Part model, mm, in its own coordinate system. Face numbers are marked on the shaded views. A direction names the side the tool comes from. Give positions to 0.01 mm unless a question says otherwise; leave off trailing zeros. Order: outer loops, then holes, each group sorted by start corner. A loop starts at its lowest first (then second) coordinate and runs counter-clockwise, first axis right, second up. Notation, with made-up numbers: M 4.5,67.5 L 45.5,67.5 A26 ccw 45.5,99.5 Z; hole C 88.5,74.5 d6. An arc over 180 degrees is marked long. One line per question, with ' | ' between items.
Autodesk Inventor part; units mm, degrees
ref_plane "YZ Plane" through (0, 0, 0) normal (1, 0, 0) x (0, 1, 0)
ref_plane "XZ Plane" through (0, 0, 0) normal (0, 1, 0) x (-1, 0, 0)
ref_plane "XY Plane" through (0, 0, 0) normal (0, 0, 1) x (1, 0, 0)
sketch "Sketch1" plane through (0, 0, 0) normal (0, 0, 1) x (1, 0, 0)
  arc A0 (-2.8807, 19.6399) -> (-2.8807, -19.6399) centre (0, 0) ccw
  arc A1 (131.6255, -39.3688) -> (131.6255, 39.3688) centre (137.4, 0) ccw
  line L0 (0, 0) -> (137.4, 0)
  line L1 (0, 0) -> (137.4, 0) construction
  line L2 (-2.8807, 19.6399) -> (131.6255, 39.3688)
  line L3 (-2.8807, -19.6399) -> (131.6255, -39.3688)
  arc A2 (131.9303, -37.291) -> (131.9303, 37.291) centre (137.4, 0) ccw
  line L4 (131.9303, 37.291) -> (-2.5759, 17.5621)
  arc A3 (-2.5759, 17.5621) -> (-2.5759, -17.5621) centre (0, 0) ccw
  line L5 (-2.5759, -17.5621) -> (131.9303, -37.291)
  arc A4 (131.4078, -40.8529) -> (131.4078, 40.8529) centre (137.4, 0) ccw
  line L6 (131.4078, 40.8529) -> (-3.0984, 21.124)
  arc A5 (-3.0984, 21.124) -> (-3.0984, -21.124) centre (0, 0) ccw
  line L7 (-3.0984, -21.124) -> (131.4078, -40.8529)
  dimension "d0" = 39.7
  dimension "d1" = 79.58
  dimension "d2" = 137.4
  dimension "d3" = 0
  dimension "d4" = 2.1
  dimension "d5" = 1.5
extrude "Extrusion1" add sketch "Sketch1" along normal blind 15 contours L2 A1 L3 A0 | L7 A5 L6 A4
properties part number "HTD5M 93 Belt" material "Rubber"
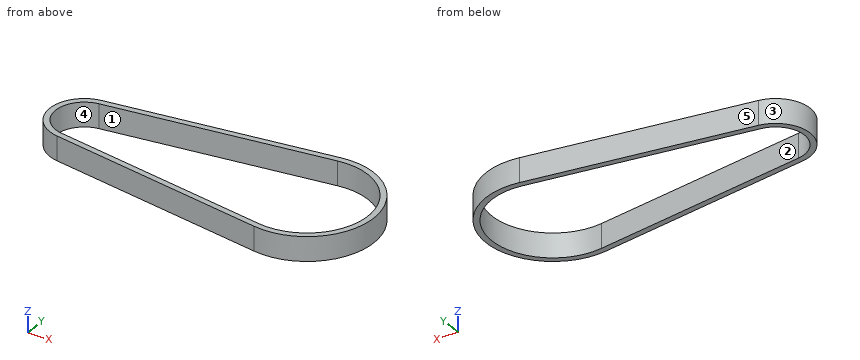
1. Slice it at A-A on x = 137.4. Give the cut face in (y, z), then the cut area to 3 significant figures.
Worked out:
outline: M -41.29,0 L -37.69,0 L -37.69,15 L -41.29,15 Z; M 37.69,0 L 41.29,0 L 41.29,15 L 37.69,15 Z | area: 108 mm2
2. Tool access for the marked faces 4 and 5: list every direction of +Z, -Z, +X, -X, +Y, -Y with a clear straight run to the whole face (end or side of a thin tool).
Worked out:
face 4: +Z, -Z | face 5: +Z, -Z, -X, +Y
3. Drop flat-ended pins along their axis: pin 1 (1 mm diameter, centred on x = 115, z = 12.5, fed in from -Y); pin 2 (6 mm diameter, centred on y = 18, z = 13, fed in from -X); pin 3 (3 mm diameter, centred on y = 23, z = 9, fed in from +X). Give the stop position or say it passes through.
Worked out:
pin 1: stops at y = -38.52 | pin 2: stops at x = -15.19 | pin 3: stops at x = 172.65
4. Mould opens along X. For the marked faces 1, 2 and 3 say: released by +X, released by -X, zero draft, split by the parting line, or undercut.
Worked out:
face 1: undercut | face 2: undercut | face 3: released by -X
5. Probe L1, parallel to Y at x = 137.4, z = 9; L2, parallel to Y at x = 88, z = 10.75; L3, parallel to X at y = 13.5, z = 6.25. List the from-to ranges inside material, lowest first. Write a range as from..to.
Worked out:
L1: y = -41.29..-37.69, 37.69..41.29 | L2: y = -34.49..-30.85, 30.85..34.49 | L3: x = -16.54..-11.52, 172.59..176.42
6. Slice it at B-B on y = 0. Give the cut face in (x, z), then the cut area to 3 significant figures.
Worked out:
outline: M -21.35,0 L -17.75,0 L -17.75,15 L -21.35,15 Z; M 175.09,0 L 178.69,0 L 178.69,15 L 175.09,15 Z | area: 108 mm2
7. Slice it at C-C on z = 11. Give the cut face in (x, y), then the cut area to 3 significant figures.
Worked out:
outline: M -3.1,-21.12 L 131.41,-40.85 A41.29 ccw long 131.41,40.85 L -3.1,21.12 A21.35 ccw Z; hole M -2.58,-17.56 L 131.93,-37.29 A37.69 ccw long 131.93,37.29 L -2.58,17.56 A17.75 ccw Z | area: 1,670 mm2
